The listing builds one solid part. Answer for the finished solid, in the listing's coordinates (mm). A direction names the side the tool comes from. Round coordinates to 2 decimals unless told otherwise and drop trailing zeros. Write each loop counter-clockwise with the first axis right and the second up, starting at its lowest first coordinate (ties: lowest second). Pieces come first, ordered by that corner, then holes. Notation, with made-up numbers: M 85,-14 L 99,-14 A25 ccw 99,20 Z; hole C 21,72.5 d4. An arc over 180 degrees is marked long. One line per item, written item: value. Start each with the question number.
(1) Section B-B (z = 0) is taken. Determine the outline of the cut face in (x, y) (3 decimals).
(2) Section C-C (z = 5.75) is taken. Determine the outline of the cut face in (x, y), plus the area to 3 significant figures.
(3) Section A-A (x = 0) is taken. Determine the outline of the cut face in (y, z) (3 decimals), plus the area to 3 significant figures.
(4) Consider probe 1 along X at (y, z) = (28.5, 5.75); probe 2 along Y at (x, z) = (-6.5, -4); probe 3 along Y at (x, z) = (0.25, 1.25). Determine where each line is inside the solid, lowest interval first.
(5) Section D-D (y = 19.5) is taken. Determine the outline of the cut face in (x, z).
(6) For faces 1 (the cylindrical face through (1, -7, 0)), 2 (the flat face through (0, 37.65, 0)), 3 (the cylindrical face through (-3, 31.29, -0.67)), determine the directions among +Z, -Z, +X, -X, +Y, -Y from which every point of the face is accessible in a straight line to the end or side of a thin tool.
(7) For a pull along X with two mould halves and no side action, classify faces 4 (the flat face through (0, 25.5, 6)), 5 (the cylindrical face through (-1, 35, 0)), 6 (the flat face through (-4.2, 0, -0.2)) as released by +X, released by -X, zero draft, split by the parting line, or undercut.
(8) Given P1, Ø10, axis at x = 1.5, y = 29.5, coming from the +Z side; P2, Ø2.5, axis at x = -0.5, z = 6.5, coming from the +Y side; P3, Ø5.5, axis at x = 4.5, z = 2.5, coming from the -Y side; P4, Ø1.5, axis at x = 0.5, z = -6, coming from the +Y side, each flat-ended and moving along its own axis, determine where each tip first touches the part or whether it passes through.
```python
from build123d import *

# Parameters (mm, degrees)
BOSS_EXTRUDE1_DEPTH = 30.5
SKETCH2_R           = 3.075
SKETCH2_R_2         = 1
BOSS_EXTRUDE2_DEPTH = 1.6
SKETCH2_2_R         = 1
BOSS_EXTRUDE3_DEPTH = 7.15
BOSS_EXTRUDE4_START = 2
SKETCH3_R           = 4
SKETCH3_R_2         = 1
BOSS_EXTRUDE4_DEPTH = 2
BOSS_EXTRUDE5_START = 12
SKETCH3_2_R         = 1
BOSS_EXTRUDE5_DEPTH = 12
SKETCH4_R           = 1.5
CUT_EXTRUDE1_DEPTH  = 5


with BuildPart() as part:
    # Sketch1 → Boss-Extrude1 (new body)
    with BuildSketch(Plane(origin=(0, 0, 0), x_dir=(1, 0, 0), z_dir=(0, 1, 0))):
        with BuildLine():
            Line((-9.15, 7.917543811), (-9.15, -7.917543811))
            ThreePointArc((-9.15, -7.917543811), (0, -12.1), (9.15, -7.917543811))
            Line((9.15, -7.917543811), (9.15, 7.917543811))
            ThreePointArc((9.15, 7.917543811), (0, 12.1), (-9.15, 7.917543811))
        make_face()
    extrude(amount=BOSS_EXTRUDE1_DEPTH)

    # Sketch2 → Boss-Extrude2 (add)
    with BuildSketch(Plane(origin=(0, 30.5, 0), x_dir=(1, 0, 0), z_dir=(0, 1, 0))):
        with Locations(Location((0, 0, 0), (0, 0, 270))):
            Circle(SKETCH2_R)
        with Locations(Location((0, 0, 0), (0, 0, 270))):
            Circle(SKETCH2_R_2, mode=Mode.SUBTRACT)
    extrude(amount=BOSS_EXTRUDE2_DEPTH)

    # Sketch2_2 → Boss-Extrude3 (add)
    with BuildSketch(Plane(origin=(0, 30.5, 0), x_dir=(1, 0, 0), z_dir=(0, 1, 0))):
        with Locations(Location((0, 0, 0), (0, 0, 270))):
            Circle(SKETCH2_2_R)
    extrude(amount=BOSS_EXTRUDE3_DEPTH)

    # Sketch3 → Boss-Extrude4 (add)
    with BuildSketch(Plane.XZ.offset(BOSS_EXTRUDE4_START)):
        with Locations(Location((0, 0, 0), (0, 0, 270))):
            Circle(SKETCH3_R)
        with Locations(Location((0, 0, 0), (0, 0, 90))):
            Circle(SKETCH3_R_2, mode=Mode.SUBTRACT)
    extrude(amount=-BOSS_EXTRUDE4_DEPTH)

    # Sketch3_2 → Boss-Extrude5 (add)
    with BuildSketch(Plane.XZ.offset(BOSS_EXTRUDE5_START)):
        with Locations(Location((0, 0, 0), (0, 0, 90))):
            Circle(SKETCH3_2_R)
    extrude(amount=-BOSS_EXTRUDE5_DEPTH)

    # Sketch4 → Cut-Extrude1 (cut)
    with BuildSketch(Plane(origin=(0, 30.5, 0), x_dir=(1, 0, 0), z_dir=(0, 1, 0))):
        with Locations(Location((0, 5.75, 0), (0, 0, 270))):
            Circle(SKETCH4_R)
        with Locations(Location((0, -5.75, 0), (0, 0, 270))):
            Circle(SKETCH4_R)
    extrude(amount=-CUT_EXTRUDE1_DEPTH, mode=Mode.SUBTRACT)


solid = part.part
```
Recorded:
1. outline: M -9.15,0 L -4,0 L -4,-2 L -1,-2 L -1,-12 L 1,-12 L 1,-2 L 4,-2 L 4,0 L 9.15,0 L 9.15,30.5 L 3.075,30.5 L 3.075,32.1 L 1,32.1 L 1,37.65 L -1,37.65 L -1,32.1 L -3.075,32.1 L -3.075,30.5 L -9.15,30.5 Z
2. outline: M -9.15,0 L 9.15,0 L 9.15,30.5 L 1.5,30.5 L 1.5,25.5 L -1.5,25.5 L -1.5,30.5 L -9.15,30.5 Z
2. area: 543 mm2
3. outline: M -12,-1 L -2,-1 L -2,-4 L 0,-4 L 0,-12.1 L 30.5,-12.1 L 30.5,-7.25 L 25.5,-7.25 L 25.5,-4.25 L 30.5,-4.25 L 30.5,-3.075 L 32.1,-3.075 L 32.1,-1 L 37.65,-1 L 37.65,1 L 32.1,1 L 32.1,3.075 L 30.5,3.075 L 30.5,4.25 L 25.5,4.25 L 25.5,7.25 L 30.5,7.25 L 30.5,12.1 L 0,12.1 L 0,4 L -2,4 L -2,1 L -12,1 Z
3. area: 765 mm2
4. probe 1: x = -9.15 to -1.5, 1.5 to 9.15
4. probe 2: y = 0 to 30.5
4. probe 3: y = -2 to 32.1
5. outline: M -9.15,-7.92 A12.1 ccw 9.15,-7.92 L 9.15,7.92 A12.1 ccw -9.15,7.92 Z
6. face 1: -Y
6. face 2: +Z, -Z, +X, -X, +Y
6. face 3: +Y
7. face 4: undercut
7. face 5: split by the parting line
7. face 6: zero draft
8. P1: stops at z = 12.1
8. P2: stops at y = 30.5
8. P3: stops at y = -2
8. P4: stops at y = 25.5
